from build123d import *

# Parameters (mm, degrees)
BOSS_EXTRU_1_DEPTH      = 50
ENL_V_START             = -13.000137383
ENL_V_MAT_EXTRU_1_DEPTH = 20.000137383


# Read off the part's stored shape, not the designer's step: Enlèv. mat.-Extru.1
with BuildPart() as part:
    # Esquisse1 → Boss.-Extru.1 (new body)
    with BuildSketch(Plane.XY.offset(-25)):
        with BuildLine():
            Line((-2, -28.65), (-2, -9.797958971))
            ThreePointArc((-2, -9.797958971), (-7.745966692, -6.32455532), (-10, 0))
            add(Edge.make_bspline(
                [(-10, 0), (-10.038102543, -9.915248827), (-2.132148039, -18.010708935), (-2, -28.65)],
                knots=[0, 0, 0, 0, 1, 1, 1, 1], degree=3))
        make_face()
        with BuildLine():
            Line((3, -11.472816521), (3, -9.539392014))
            ThreePointArc((3, -9.539392014), (0.516443819, -9.986655385), (-2, -9.797958971))
            Line((-2, -9.797958971), (-2, -28.65))
            Line((-2, -28.65), (-2, -57.3))
            Line((-2, -57.3), (3, -57.3))
            Line((3, -57.3), (3, -11.472816521))
        make_face()
        with BuildLine():
            ThreePointArc((9.899806533, -1.412030667), (7.623303271, -6.471881275), (3, -9.539392014))
            Line((3, -9.539392014), (3, -11.472816521))
            add(Edge.make_bspline(
                [(9.899806533, -1.412030667), (9.042464712, -8.684319248), (3.317345852, -8.787272714), (3, -11.472816521)],
                knots=[0.05745519, 0.05745519, 0.05745519, 0.05745519, 1, 1, 1, 1], degree=3))
        make_face()
        with BuildLine():
            ThreePointArc((-2, -1.5), (-0.790569415, 2.371708245), (2.5, 0))
            Line((2.5, 0), (3, 0))
            Line((3, 0), (3, -9.539392014))
            ThreePointArc((3, -9.539392014), (7.623303271, -6.471881275), (9.899806533, -1.412030667))
            add(Edge.make_bspline(
                [(10, 0), (9.986241611, -0.498789425), (9.952067961, -0.968730021), (9.899806533, -1.412030667)],
                knots=[0, 0, 0, 0, 0.05745519, 0.05745519, 0.05745519, 0.05745519], degree=3))
            ThreePointArc((10, 0), (0, 10), (-10, 0))
            ThreePointArc((-10, 0), (-7.745966692, -6.32455532), (-2, -9.797958971))
            Line((-2, -9.797958971), (-2, -1.5))
        make_face()
        with BuildLine():
            Line((3, 0), (2.5, 0))
            ThreePointArc((2.5, 0), (0.790569415, -2.371708245), (-2, -1.5))
            Line((-2, -1.5), (-2, -9.797958971))
            ThreePointArc((-2, -9.797958971), (0.516443819, -9.986655385), (3, -9.539392014))
            Line((3, -9.539392014), (3, 0))
        make_face()
    extrude(amount=BOSS_EXTRU_1_DEPTH)

    # Enlèv. mat.-Extru.1 outline → Enlèv. mat.-Extru.1 (cut)
    with BuildSketch(Plane(origin=(3, 0, 0), x_dir=(0, 0, -1), z_dir=(1, 0, 0)).offset(ENL_V_START)):
        with BuildLine():
            Line((-25, -57.3), (-10, -57.3))
            Line((-10, -57.3), (-10, -37.083079187))
            add(Edge.make_bspline(
                [(-10, -37.083079187), (-10.308820918, -33.626949696), (-24.959081539, -27.805521116), (-25, -20.002816521)],
                knots=[0.33438903, 0.33438903, 0.33438903, 0.33438903, 1.313600201, 1.313600201, 1.313600201, 1.313600201], degree=3))
            Line((-25, -20.002816521), (-25, -57.3))
        make_face()
        with BuildLine():
            Line((10, -37.3), (10, -57.3))
            Line((10, -57.3), (25, -57.3))
            Line((25, -57.3), (25, -20.310673404))
            add(Edge.make_bspline(
                [(25, -20.310673404), (24.825306853, -28.916467162), (10.047414043, -34.103142781), (10, -37.3)],
                knots=[0.656671032, 0.656671032, 0.656671032, 0.656671032, 1.644941889, 1.644941889, 1.644941889, 1.644941889], degree=3))
        make_face()
        with BuildLine():
            add(Edge.make_bspline(
                [(0.174087167, -33.300000001), (8.510773732, -33.241503729), (20.989133498, -24.836380481), (20.999995082, -20.00281651)],
                knots=[0.00693536, 0.00693536, 0.00693536, 0.00693536, 0.999807124, 0.999807124, 0.999807124, 0.999807124], degree=3))
            Line((20.999995082, -20.00281651), (21, 10.000000033))
            Line((21, 10.000000033), (-21, 10))
            Line((-21, 10), (-21.000000005, -20.035970331))
            add(Edge.make_bspline(
                [(0, -33.3), (-12.278821067, -33.266087617), (-20.974999639, -24.210992728), (-21.000000005, -20.035970331)],
                knots=[0, 0, 0, 0, 0.99712668, 0.99712668, 0.99712668, 0.99712668], degree=3))
            Line((0, -33.3), (0.174087167, -33.300000001))
        make_face()
    extrude(amount=ENL_V_MAT_EXTRU_1_DEPTH, mode=Mode.SUBTRACT)


solid = part.part
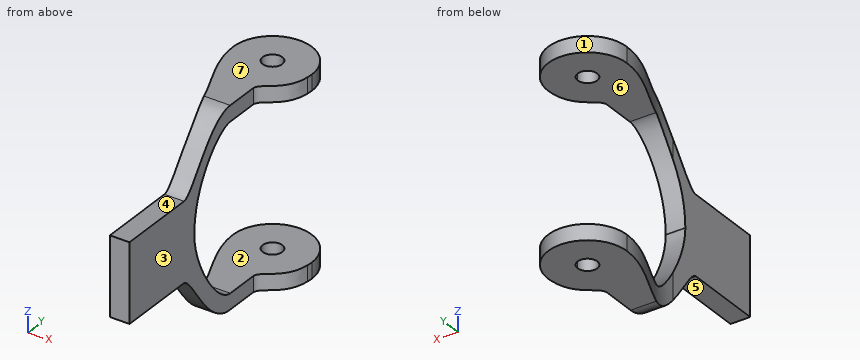
Geometry: final body of the model. Coordinates: model frame, mm. Face numbers are marked on the shaded views. A direction names the side the tool comes from. Give positions to 0.01 mm unless a question says otherwise; leave off trailing zeros. Write each loop counter-clockwise with the first axis right and the second up, starting at its lowest first coordinate (ties: lowest second). Pieces come first, ordered by that corner, then holes. Notation, with made-up numbers: (71, 0) -> (76, 0) arc R25 ccw to (76, 39) -> close; hole circle Ø8 at (35, 4.25). An arc over 180 degrees is marked (long way). Answer in a Markdown table with one row per item.
(1) Ray query, line 1 along Z through (x, y) = (8.25, -5); line 2 along Z through (x, y) = (-1, -26); line 3 along Z through (x, y) = (1.25, -45). Return the intervals inside material, ascending. Write a range as [from, to].
Answers below:
| item | result |
|---|---|
| line 1 | [-25, -21], [21, 25] |
| line 2 | [-22.71, -16.98], [17.64, 22.24] |
| line 3 | [-10, 10] |
(2) Section query A-A on y = 6. Return loops of the section in (x, z), then the cut area to 3 significant figures.
Answers below:
| item | result |
|---|---|
| outline | (-8, -25) -> (8, -25) -> (8, -21) -> (-8, -21) -> close; (-8, 21) -> (8, 21) -> (8, 25) -> (-8, 25) -> close |
| area | 128 mm^2 |
(3) Section query C-C on y = -39. Return loops of the section in (x, z).
Answers below:
| item | result |
|---|---|
| outline | (-2, -10) -> (3, -10) -> (3, 10) -> (-2, 10) -> close |
(4) Section query B-B on x = 0. State how many separate pieces and enclosed holes the cut face has, then the cut area to 3 significant figures.
Answers below:
| item | result |
|---|---|
| separate pieces | 3 |
| enclosed holes | 0 |
| area | 846 mm^2 |
(5) Pin query (flat end, axial travel): pin 1 (23 mm diameter, centred on y = -41, z = -9.5, fed in from +X); pin 2 (4 mm diameter, centred on x = 1.5, y = -44, fed in from -Z); pin 3 (6 mm diameter, centred on x = -4.5, y = -47.5, fed in from +Z). Return the tip coordinate at first contact, or that it passes through.
Answers below:
| item | result |
|---|---|
| pin 1 | x = 3 |
| pin 2 | z = -10 |
| pin 3 | z = 10 |
(6) Draft query along Z for the marked faces 5, 6 and 7. Return one class per face: +Z half, -Z half, draft (parallel to the pull), parting line (faces both ways), or undercut.
Answers below:
| item | result |
|---|---|
| face 5 | -Z half |
| face 6 | undercut |
| face 7 | +Z half |
(7) Set-up query: the marked faces 1, 2, 3 and 4. Return all of +Z, -Z, +X, -X, +Y, -Y with unobstructed straight access to the full face (end or side cutting, diameter ignored); none if empty.
Answers below:
| item | result |
|---|---|
| face 1 | +Z, -Z, +Y |
| face 2 | +X, -X, +Y |
| face 3 | +Z, -Z, +X, -Y |
| face 4 | +Z, +X, -X, -Y |
